from build123d import *

# Parameters (mm, degrees)
SKETCH_1_R          = 20
SKETCH_1_R_2        = 15
EXTRUDE_1_DEPTH     = 3
SKETCH_2_R          = 2.5
CUT_EXTRUDE_1_DEPTH = 92.262525064


with BuildPart() as part:
    # 草图1 → 凸台-拉伸1 (new body)
    with BuildSketch(Plane(origin=(0, 0, 0), x_dir=(1, 0, 0), z_dir=(0, 1, 0))):
        Circle(SKETCH_1_R)
        with BuildLine():
            ThreePointArc((20, 0), (8.309115435, -18.192267607), (-13.095860068, -15.116165158))
            Line((-13.095860068, -15.116165158), (39.675579632, -60.834598551))
            ThreePointArc((39.675579632, -60.834598551), (38.890872965, -38.890872965), (60.834598551, -39.675579632))
            Line((60.834598551, -39.675579632), (15.116165158, 13.095860068))
            ThreePointArc((15.116165158, 13.095860068), (18.73930766, 6.98844392), (20, 0))
        make_face()
        with Locations((49.497474683, -49.497474683)):
            Circle(SKETCH_1_R_2)
    extrude(amount=EXTRUDE_1_DEPTH)

    # 草图2 → 切除-拉伸1 (cut, through all)
    with BuildSketch(Plane(origin=(0, 3, 0), x_dir=(1, 0, 0), z_dir=(0, 1, 0))):
        with Locations(Location((0, 0, 0), (0, 0, 270))):
            Circle(SKETCH_2_R)
    extrude(amount=-CUT_EXTRUDE_1_DEPTH, mode=Mode.SUBTRACT)


solid = part.part
For this review, take the finished solid that the model builds, in its own axes (mm). Round coordinates to 2 decimals unless told otherwise and drop trailing zeros. Write each loop counter-clockwise with the first axis right and the second up, starting at its lowest first coordinate (ties: lowest second). Pieces come first, ordered by that corner, then holes. Notation, with made-up numbers: (77.25, 41) - (109.25, 41) arc R28 ccw to (109.25, 59) - close; hole circle Ø10 at (-35, 47.5). An arc over 180 degrees is marked (long way). Write item = value, one per line. Start each with the question number.
1. Draft analysis for pull direction Z (two halves, no side actions). For faces 1 (the face through (38.295, 1.479, 13.659)), 2 (the face through (-2.44, 1.52, -0.54)), 3 (the face through (-13.813, 1.479, -14.464)), state which applies: released by +Z, released by -Z, zero draft, split by the parting line, or undercut.
2. Consider section B-B on y = 0.5. State the section outline as (x, z) points, plus the area to 3 significant figures.
3. Consider section C-C on z = 0. State the section outline as (x, y) points, plus the area to 3 significant figures.
4. Consider section A-A on x = 0. State the section outline as (y, z) points.
5. Consider section D-D on x = 17.5. State the section outline as (y, z) points.
6. Wall thickness on L1, parallel to X at y = 2, z = -0.5; L2, parallel to X at y = 2.2, z = 0; L3, parallel to Z at x = 54, y = 1.35: over which ranges is each line inside the solid? List them lowest first.
Evaluation:
q1.face_1 = released by -Z
q1.face_2 = undercut
q1.face_3 = split by the parting line
q2.outline = (-13.1, 15.12) arc R20 ccw (long way) to (15.12, -13.1) - (60.83, 39.68) arc R15 ccw to (39.68, 60.83) - close; hole circle Ø5 at (0, 0)
q2.area = 3,420 mm2
q3.outline = (-20, 0) - (-2.5, 0) - (-2.5, 3) - (-20, 3) - close; (2.5, 0) - (26.46, 0) - (26.46, 3) - (2.5, 3) - close
q3.area = 124 mm2
q4.outline = (0, -20) - (3, -20) - (3, -2.5) - (0, -2.5) - close; (0, 2.5) - (3, 2.5) - (3, 26.46) - (0, 26.46) - close
q5.outline = (0, -10.34) - (3, -10.34) - (3, 41.62) - (0, 41.62) - close
q6.L1 = -19.99 to -2.45, 2.45 to 26.03
q6.L2 = -20 to -2.5, 2.5 to 26.46
q6.L3 = 31.79 to 63.81
